The listing builds one solid part. Answer for the finished solid, in the listing's coordinates (mm). Round coordinates to 2 decimals unless told otherwise and drop trailing zeros. Order: outer loops, then holes, each group sorted by start corner. A loop starts at its lowest first (then second) coordinate and runs counter-clockwise, first axis right, second up. Notation, with made-up numbers: (-18, 46.25) - (28, 46.25) arc R32 cw to (28, 79.25) - close; hole circle Ø3 at (75.5, -33.5). An arc over 180 degrees is marked (long way). Use CSV: the item, a comma, the result in double quotes. Start each with the question number.
Item 1: Find section A-A, the plane z = 0. Give the vertices of the cut face in (x, y).
Item 2: Find section B-B, the plane y = 271.5. Give the vertices of the cut face in (x, z), plus the area to 3 significant figures.
Item 3: Find section C-C, the plane x = 8.5. Give the vertices of the cut face in (y, z), plus the area to 3 significant figures.
Item 4: Straight lines are drawn through the part: line 1 along Y through (x, z) = (9.5, 3); line 2 along Y through (x, z) = (0.75, -9); line 3 along Z through (x, y) = (-0.5, 147). For each, find the intervals that lie inside material, in ascending order. Write a range as [from, to].
Item 5: Flat-ended cylindrical pins translate along their axes: P1, Ø12, axis at x = 9, z = 1, coming from the +Y side; P2, Ø6, axis at y = 351, z = 7.5, coming from the +X side; P3, Ø5, axis at y = 101, z = 6, coming from the -X side. Find the tip coordinate at first contact, or state that the pin passes through.
Autodesk Inventor part; units mm, degrees
ref_plane "YZ Plane" through (0, 0, 0) normal (1, 0, 0) x (0, 1, 0)
ref_plane "XZ Plane" through (0, 0, 0) normal (0, 1, 0) x (-1, 0, 0)
ref_plane "XY Plane" through (0, 0, 0) normal (0, 0, 1) x (1, 0, 0)
sketch "Sketch1" plane through (0, 0, 0) normal (0, 1, 0) x (-1, 0, 0)
  circle A0 centre (0, 0) radius 13.5
  dimension "d0" = 27
extrude "Extrusion1" add sketch "Sketch1" along normal blind 436
sketch "Sketch2" plane through (0, 436, 0) normal (0, 1, 0) x (1, 0, 0)
  circle A0 centre (0, -8.8) radius 1
  circle A1 centre (0, 8.8) radius 1
  circle A2 centre (0, 0) radius 13.5
  dimension "d3" = 2
  dimension "d4" = 2
  dimension "d5" = 8.8
  dimension "d6" = 8.8
extrude "Extrusion2" add sketch "Sketch2" along normal blind 7 contours A0 | A1
sketch "Sketch3" plane through (0, 0, 0) normal (0, -1, 0) x (1, 0, 0)
  circle A0 centre (0, 8) radius 1
  circle A1 centre (0, -8) radius 1
  point P0 (0, 0)
  dimension "d9" = 2
  dimension "d10" = 2
  dimension "d15" = 8
  dimension "d16" = 8
extrude "Extrusion3" add sketch "Sketch3" along normal blind 7
sketch "Sketch4" plane through (0, 0, 0) normal (0, -1, 0) x (1, 0, 0)
  point P0 (0, 0)
properties part number "UV-15W"
Worked out:
1,outline,"(-13.5, 0) - (13.5, 0) - (13.5, 436) - (-13.5, 436) - close"
2,outline,"circle Ø27 at (0, 0)"
2,area,"573 mm²"
3,outline,"(0, -10.49) - (436, -10.49) - (436, 10.49) - (0, 10.49) - close"
3,area,"9,150 mm²"
4,line 1,"y = [0, 436]"
4,line 2,"y = [0, 443]"
4,line 3,"z = [-13.49, 13.49]"
5,P1,"stops at y = 436"
5,P2,"stops at x = 12.73"
5,P3,"stops at x = -13.04"
